from build123d import *

# Parameters (mm, degrees)
F0_R     = 6.35
F1_DEPTH = 6.35


with BuildPart() as f1:
    # F0 (on Front) → F1 (new body)
    with BuildSketch(Plane.XZ):
        Polygon((44.196, 27.94), (37.846, 27.94), (34.925, 27.94), (34.925, 34.29), (28.575, 34.29), (28.575, 27.94), (22.225, 27.94), (22.225, 34.29), (15.875, 34.29), (15.875, 27.94), (9.525, 27.94), (9.525, 34.29), (3.175, 34.29), (3.175, 27.94), (-3.175, 27.94), (-3.175, 34.29), (-9.525, 34.29), (-9.525, 27.94), (-15.875, 27.94), (-15.875, 34.29), (-22.225, 34.29), (-22.225, 27.94), (-28.575, 27.94), (-28.575, 34.29), (-34.925, 34.29), (-34.925, 27.94), (-37.846, 27.94), (-44.196, 27.94), (-44.196, 22.225), (-37.846, 22.225), (-37.846, 15.875), (-44.196, 15.875), (-44.196, 9.525), (-37.846, 9.525), (-37.846, 3.175), (-44.196, 3.175), (-44.196, -3.175), (-37.846, -3.175), (-37.846, -9.525), (-44.196, -9.525), (-44.196, -15.875), (-37.846, -15.875), (-37.846, -22.225), (-44.196, -22.225), (-44.196, -27.94), (-37.846, -27.94), (-34.925, -27.94), (-34.925, -34.29), (-28.575, -34.29), (-28.575, -27.94), (-22.225, -27.94), (-22.225, -34.29), (-15.875, -34.29), (-15.875, -27.94), (-9.525, -27.94), (-9.525, -34.29), (-3.175, -34.29), (-3.175, -27.94), (3.175, -27.94), (3.175, -34.29), (9.525, -34.29), (9.525, -27.94), (15.875, -27.94), (15.875, -34.29), (22.225, -34.29), (22.225, -27.94), (28.575, -27.94), (28.575, -34.29), (34.925, -34.29), (34.925, -27.94), (37.846, -27.94), (44.196, -27.94), (44.196, -22.225), (37.846, -22.225), (37.846, -15.875), (44.196, -15.875), (44.196, -9.525), (37.846, -9.525), (37.846, -3.175), (44.196, -3.175), (44.196, 3.175), (37.846, 3.175), (37.846, 9.525), (44.196, 9.525), (44.196, 15.875), (37.846, 15.875), (37.846, 22.225), (44.196, 22.225), align=None)
        with Locations((0, 3.81)):
            Circle(F0_R, mode=Mode.SUBTRACT)
    extrude(amount=F1_DEPTH)


solid = f1.part
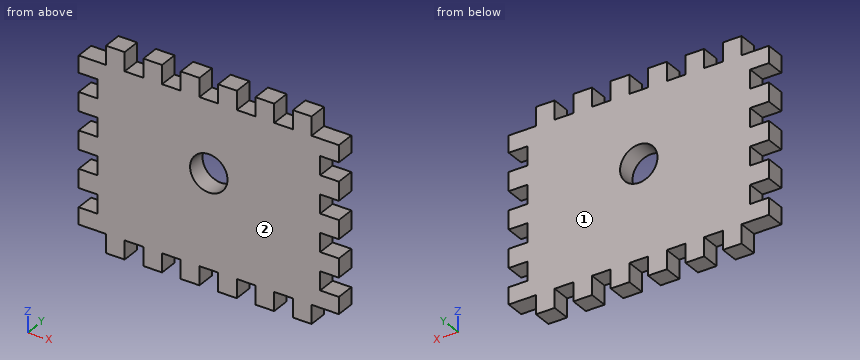
The model under review builds one solid part; all positions refer to its coordinate system, in mm. Face numbers are marked on the shaded views. Round coordinates to 2 decimals unless told otherwise and drop trailing zeros. Loops run counter-clockwise (first coordinate to the right, second up) from the corner with the lowest first, then second, coordinate; pieces in that order, holes last. Notation, with made-up numbers: (33, -19) -> (91, -19) arc R14 cw to (91, -7) -> close; hole circle Ø6 at (34, 54). An arc over 180 degrees is marked (long way). One line per question, with ' | ' between items. Start each with the question number.
Item 1: Add section B-B, the plane z = -20. Write out the cut boundary in (x, y), then the cut area to 3 significant figures.
Item 2: Add section C-C, the plane x = -11. Write out the cut boundary in (y, z).
Item 3: For pin 1 (1.9 mm diameter, centred on x = 40, y = -3, fed in from -Z); pin 2 (1.5 mm diameter, centred on y = -1, z = 8, fed in from -X); pin 3 (3 mm diameter, centred on y = -3.5, z = -32.5, fed in from +X) (3 decimals); pin 4 (4 mm diameter, centred on x = -22.5, z = 4, fed in from +Y), all flat-tipped, find the tip position at first contact; note any pin that passes through.
Item 4: Add section A-A, the plane x = 0. Write out the cut boundary in (y, z).
Item 5: Wall thickness on line 1 along Z through (x, y) = (0, -1.75); line 2 along Z through (x, y) = (-4.5, -5.25); line 3 along X through (y, z) = (-2, 17): over which ranges is each line inside the solid? List them lowest first. Write a range as [from, to].
Item 6: Draft analysis for pull direction Y (two halves, no side actions). For the marked faces 1 and 2, state which applies: +Y half, -Y half, draft (parallel to the pull), parting line (faces both ways), or undercut.
Return value:
1) outline: (-37.85, -6.35) -> (37.85, -6.35) -> (37.85, 0) -> (-37.85, 0) -> close | area: 481 mm2
2) outline: (-6.35, -27.94) -> (0, -27.94) -> (0, 27.94) -> (-6.35, 27.94) -> close
3) pin 1: stops at z = -27.94 | pin 2: stops at x = -37.85 | pin 3: stops at x = 34.925 | pin 4: stops at y = 0
4) outline: (-6.35, -27.94) -> (0, -27.94) -> (0, -2.54) -> (-6.35, -2.54) -> close; (-6.35, 10.16) -> (0, 10.16) -> (0, 27.94) -> (-6.35, 27.94) -> close
5) line 1: z = [-27.94, -2.54], [10.16, 27.94] | line 2: z = [-34.29, -0.67], [8.29, 34.29] | line 3: x = [-37.85, 37.85]
6) face 1: +Y half | face 2: -Y half
